```python
from build123d import *

# Parameters (mm, degrees)
F0_R            = 21.158401666
F0_R_2          = 3.048
F1_DEPTH        = 4.064
F3_DEPTH        = 4.064
F3_COPIES_COUNT = 32


# Not quite as in the source:
# - a pattern or mirror of a feature is missing from the dataset's text; its kind, count and spacing are read off the source's solid


with BuildPart() as f1:
    # F0 (on Top) → F1 (new body)
    with BuildSketch(Plane.XY):
        Circle(F0_R)
        Circle(F0_R_2, mode=Mode.SUBTRACT)
    extrude(amount=F1_DEPTH)

    # F2 (on face) → F3 (cut, through all)
    with BuildSketch(Plane.XY.offset(4.064)):
        with BuildLine():
            Line((-0.4109729921, -18.2450008044), (-1.6185707702, -21.0964022933))
            ThreePointArc((-1.6185707702, -21.0964022933), (0, -21.158401666), (1.6185707702, -21.0964022933))
            Line((1.6185707702, -21.0964022933), (0.4109729921, -18.2450008044))
            ThreePointArc((0.4109729921, -18.2450008044), (0, -17.9727420469), (-0.4109729921, -18.2450008044))
        make_face()
    f3 = extrude(amount=-F3_DEPTH, mode=Mode.SUBTRACT)

    # F3_copies: F3 ×32 about axis
    f3_copies_axis = Axis((0, 0, 0), (0, 0, 1))
    for i in range(1, F3_COPIES_COUNT):
        add(f3.rotate(f3_copies_axis, i * 360 / F3_COPIES_COUNT), mode=Mode.SUBTRACT)


solid = f1.part
```
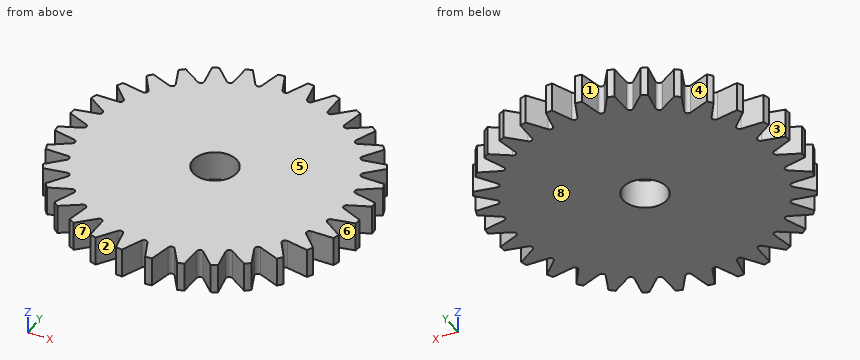
Input: part model. Units: mm. Frame: model coordinates. Face numbers are marked on the shaded views. A direction names the side the tool comes from. Give positions to 0.01 mm unless a question says otherwise; leave off trailing zeros. Order: outer loops, then holes, each group sorted by start corner. A loop starts at its lowest first (then second) coordinate and runs counter-clockwise, first axis right, second up. Notation, with made-up numbers: (15.5, 34) - (43.5, 34) arc R19 cw to (43.5, 67) - close; hole circle Ø7 at (35.5, 72). An arc over 180 degrees is marked (long way). Put each result on its own line as item: value.
Item 1: Ray query, L1, parallel to Y at x = 0, z = 3.2; L2, parallel to Y at x = 13, z = 2.5; L3, parallel to X at y = -15.5, z = 3.75. Return the intervals inside material, ascending. Write a range as from..to.
Found:
L1: y = -17.97..-3.05, 3.05..17.97
L2: y = -16.6..-14.15, -12.58..12.58, 14.15..16.6
L3: x = -13.55..-11.33, -9.81..9.81, 11.33..13.55
Item 2: Draft query along X for the marked faces 6, 7 and 8. Return one class per face: +X half, -X half, draft (parallel to the pull), parting line (faces both ways), or undercut.
Found:
face 6: +X half
face 7: undercut
face 8: draft
Item 3: Access query for the marked faces 1, 2, 3, 4 and 5. Directions: +Z, -Z, +X, -X, +Y, -Y. A direction counts if a zero-diameter tool reaches every point of the face in a straight line with its end or side. Return the directions, or none.
Found:
face 1: +Z, -Z, +Y
face 2: +Z, -Z, -Y
face 3: +Z, -Z, -X
face 4: +Z, -Z
face 5: +Z, +X, -X, +Y, -Y
Item 4: Section query B-B, the plane x = -8. Return loops of the section in (y, z), then the cut area to 3 significant figures.
Found:
outline: (-17.33, 0) - (17.33, 0) - (17.33, 4.06) - (-17.33, 4.06) - close
area: 141 mm^2
Item 5: Contact query for flat-ended pins moving along their axis: pin 1 (5.5 mm diameter, centred on x = 0, y = 0, fed in from -Z); pin 2 (2 mm diameter, centred on x = 4.5, z = 1.5, fed in from +Y). Output: stop coordinate, or through.
Found:
pin 1: passes through
pin 2: stops at y = 20.08
Item 6: Section query A-A, the plane x = 11.5. Return loops of the section in (y, z).
Found:
outline: (-15.61, 0) - (15.61, 0) - (15.61, 4.06) - (-15.61, 4.06) - close
